Part model, mm, in its own coordinate system. Face numbers are marked on the shaded views. A direction names the side the tool comes from. Coordinates: 2 decimals unless noted, no trailing zeros. Order: outer loops, then holes, each group sorted by start corner. A loop starts at its lowest first (then second) coordinate and runs counter-clockwise, first axis right, second up.
1) Wall check: L1, parallel to X at y = -1.5, z = 2; L2, parallel to Y at x = 17.5, z = 9.5; L3, parallel to X at y = -7.5, z = 10.5. Give the ranges that are in metal, low to high.
2) Cut at B-B (x = -17.5). List the corners of the cut face in (y, z), and give its area (3 significant figures).
3) Tool access for the marked faces 1 and 2: list every direction of +Z, -Z, +X, -X, +Y, -Y with a clear straight run to the whole face (end or side of a thin tool).
4) Cut at D-D (x = -9.5). List the corners of the cut face in (y, z).
5) Mould opens along X. For the marked faces 3, 4 and 5 say: +X half, -X half, draft (parallel to the pull), parting line (faces both ways), or undercut.
6) Pin check, flat tips, straight feed: pin 1 Ø1.5 at (y, z) = (-12.5, 3.5) entering from -X; pin 2 Ø1.5 at (y, z) = (-3.5, 3.5) entering from +X; pin 3 Ø5 at (y, z) = (-6, 14) entering from -X. Stop position of each tip, or through.
7) Cut at A-A (y = -0.75). List the corners of the cut face in (x, z).
8) Cut at C-C (z = 8). Give the number of separate pieces and of enclosed holes in the cut face, and give its area (3 significant figures).
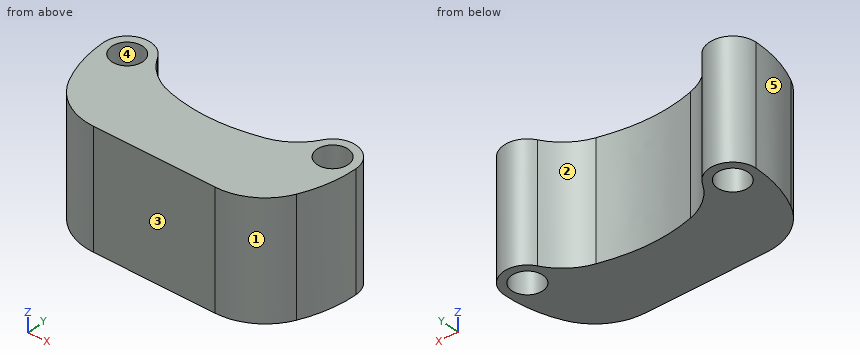
```python
from build123d import *

# Parameters (mm, degrees)
SCHIZZO1_R                   = 2.65
ESTRUSIONE_ESTRUSIONE1_DEPTH = 20
RACCORDO1_R                  = 10


with BuildPart() as part:
    # Schizzo1 → Estrusione-Estrusione1 (new body)
    with BuildSketch(Plane.XY):
        with BuildLine():
            Line((-15.402921801, -15), (15.402921801, -15))
            ThreePointArc((15.402921801, -15), (19.917490037, -8.095899619), (21.5, 0))
            ThreePointArc((21.5, 0), (18.550983955, 3.85946016), (14.052283637, 2.028115352))
            ThreePointArc((14.052283637, 2.028115352), (11.496390023, -0.853653439), (8.040859025, -2.555560913))
            add(Edge.make_bspline(
                [(-7.852499182, -2.82564864), (-5.063118639, -3.566960484), (0.144262576, -4.132980744), (5.056977543, -3.361609436), (8.040859025, -2.555560913)],
                knots=[0.170124619, 0.170124619, 0.170124619, 0.170124619, 0.505124636, 0.849602566, 0.849602566, 0.849602566, 0.849602566], degree=3))
            ThreePointArc((-7.852499182, -2.82564864), (-11.415971798, -1.060452164), (-14.009724205, 1.953963888))
            ThreePointArc((-14.009724205, 1.953963888), (-18.509677379, 3.870471753), (-21.5, 0))
            ThreePointArc((-21.5, 0), (-19.917490037, -8.095899619), (-15.402921801, -15))
        make_face()
        with Locations(Location((-17.5, 0, 0), (0, 0, 180))):
            Circle(SCHIZZO1_R, mode=Mode.SUBTRACT)
        with Locations(Location((17.5, 0, 0), (0, 0, 180))):
            Circle(SCHIZZO1_R, mode=Mode.SUBTRACT)
    extrude(amount=ESTRUSIONE_ESTRUSIONE1_DEPTH)

    # Raccordo1
    raccordo1_edges = [part.edges().sort_by_distance(p)[0] for p in [
        (15.402921801, -15, 10),
        (-15.402921801, -15, 10),
    ]]
    fillet(raccordo1_edges, radius=RACCORDO1_R)


solid = part.part
```
Geometry check:
1. L1: x = -21.45 to -19.68, -15.32 to -10.8, 10.54 to 15.32, 19.68 to 21.45
1. L2: y = -12 to -2.65, 2.65 to 4
1. L3: x = -20.15 to 20.15
2. outline: (-12, 0) - (-2.65, 0) - (-2.65, 20) - (-12, 20) - close; (2.65, 0) - (4, 0) - (4, 20) - (2.65, 20) - close
2. area: 214 mm2
3. face 1: +Z, -Z, +X, -Y
3. face 2: +Z, -Z, +Y
4. outline: (-15, 0) - (-2.23, 0) - (-2.23, 20) - (-15, 20) - close
5. face 3: draft
5. face 4: undercut
5. face 5: -X half
6. pin 1: stops at x = -17.73
6. pin 2: stops at x = 21.32
6. pin 3: stops at x = -21.21
7. outline: (-21.49, 0) - (-20.04, 0) - (-20.04, 20) - (-21.49, 20) - close; (-14.96, 0) - (-11.8, 0) - (-11.8, 20) - (-14.96, 20) - close; (11.63, 0) - (14.96, 0) - (14.96, 20) - (11.63, 20) - close; (20.04, 0) - (21.49, 0) - (21.49, 20) - (20.04, 20) - close
8. separate pieces: 1
8. enclosed holes: 2
8. area: 517 mm2
